from build123d import *

# Parameters (mm, degrees)
SKETCH1_R                = 50
BOSS_EXTRUDE1_DEPTH      = 70
BOSS_EXTRUDE2_REACH      = 223.642
BOSS_EXTRUDE2_END_RADIUS = 65
SKETCH2_R                = 42
SKETCH3_R                = 39.5
BOSS_EXTRUDE3_DEPTH      = 1
SKETCH6_R                = 41.25
BOSS_EXTRUDE4_DEPTH      = 1
BOSS_EXTRUDE5_START      = 7
SKETCH7_R                = 42
BOSS_EXTRUDE5_DEPTH      = 7
SKETCH8_R                = 35
BOSS_EXTRUDE6_DEPTH      = 3
SKETCH9_R                = 2.25
SKETCH9_R_2              = 1.5
BOSS_EXTRUDE8_DEPTH      = 1
CIRPATTERN1_COUNT        = 16
SKETCH10_R               = 10
BOSS_EXTRUDE9_DEPTH      = 10


with BuildPart() as part:
    # Sketch1 → Boss-Extrude1 (new, symmetric)
    with BuildSketch(Plane.XY):
        with BuildLine():
            Line((-80, -40), (-80, 40))
            Line((-80, 40), (-22.281665693, 61.061668614))
            ThreePointArc((-22.281665693, 61.061668614), (65, 0), (-22.281665693, -61.061668614))
            Line((-22.281665693, -61.061668614), (-80, -40))
        make_face()
        Circle(SKETCH1_R, mode=Mode.SUBTRACT)
    extrude(amount=BOSS_EXTRUDE1_DEPTH, both=True)

    # Boss-Extrude2: up to this cylinder (the profile starts outside it)
    boss_extrude2_end = Plane(origin=(0, 0, 0), z_dir=(0, 0, -1)) * Cylinder(BOSS_EXTRUDE2_END_RADIUS, 578.284, mode=Mode.PRIVATE)
    # Sketch2 → Boss-Extrude2 (add, up to the surface)
    with BuildSketch(Plane(origin=(120, 0, 0), x_dir=(0, 0, -1), z_dir=(1, 0, 0)), mode=Mode.PRIVATE) as boss_extrude2_sk1:
        Circle(SKETCH2_R)
    boss_extrude2_tool1 = extrude(boss_extrude2_sk1.sketch, amount=-BOSS_EXTRUDE2_REACH, mode=Mode.PRIVATE) - boss_extrude2_end
    add(boss_extrude2_tool1.solids().sort_by_distance((120, 0, 0))[0])

    # Sketch3 → Boss-Extrude3 (add)
    with BuildSketch(Plane(origin=(120, 0, 0), x_dir=(0, 0, -1), z_dir=(1, 0, 0))):
        Circle(SKETCH3_R)
    extrude(amount=BOSS_EXTRUDE3_DEPTH)

    # Sketch5 → Revolve1 (revolve)
    with BuildSketch(Plane.XY, mode=Mode.PRIVATE) as revolve1_sk:
        with BuildLine():
            Line((121, 0), (121, 40))
            ThreePointArc((121, 40), (131, 41.376973739), (141, 40))
            Line((141, 40), (141, 0))
            Line((141, 0), (121, 0))
        make_face()
    revolve(revolve1_sk.sketch.rotate(Axis((121, 0, 0), (1, 0, 0)), 90), axis=Axis((121, 0, 0), (1, 0, 0)))

    # Sketch6 → Boss-Extrude4 (add)
    with BuildSketch(Plane(origin=(141, 0, 0), x_dir=(0, 0, -1), z_dir=(1, 0, 0))):
        Circle(SKETCH6_R)
    extrude(amount=BOSS_EXTRUDE4_DEPTH)

    # Sketch7 → Boss-Extrude5 (add)
    with BuildSketch(Plane(origin=(142, 0, 0), x_dir=(0, 0, -1), z_dir=(1, 0, 0)).offset(BOSS_EXTRUDE5_START)):
        Circle(SKETCH7_R)
    boss_extrude5 = extrude(amount=-BOSS_EXTRUDE5_DEPTH)

    # Sketch8 → Boss-Extrude6 (add)
    with BuildSketch(Plane(origin=(149, 0, 0), x_dir=(0, 0, -1), z_dir=(1, 0, 0))):
        Circle(SKETCH8_R)
    extrude(amount=BOSS_EXTRUDE6_DEPTH)

    # Sketch9 → Boss-Extrude8 (add)
    with BuildSketch(Plane(origin=(149, 0, 0), x_dir=(0, 0, -1), z_dir=(1, 0, 0))):
        with Locations((38.5, 0)):
            Circle(SKETCH9_R)
        with Locations((38.5, 0)):
            Circle(SKETCH9_R_2, mode=Mode.SUBTRACT)
    boss_extrude8 = extrude(amount=BOSS_EXTRUDE8_DEPTH)

    # CirPattern1: Boss-Extrude5, Boss-Extrude8 ×16 about axis
    cirpattern1_axis = Axis((0, 0, 0), (1, 0, 0))
    add([boss_extrude5.rotate(cirpattern1_axis, i * 360 / CIRPATTERN1_COUNT) for i in range(1, CIRPATTERN1_COUNT)])
    add([boss_extrude8.rotate(cirpattern1_axis, i * 360 / CIRPATTERN1_COUNT) for i in range(1, CIRPATTERN1_COUNT)])

    # Sketch10 → Boss-Extrude9 (add)
    with BuildSketch(Plane(origin=(152, 0, 0), x_dir=(0, 0, -1), z_dir=(1, 0, 0))):
        Circle(SKETCH10_R)
    extrude(amount=BOSS_EXTRUDE9_DEPTH)


solid = part.part
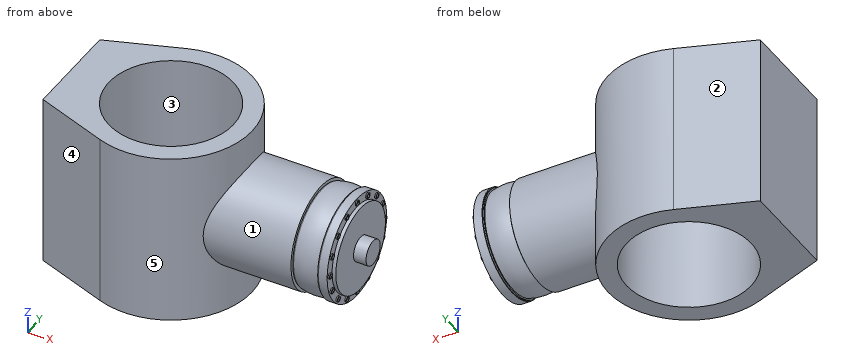
Part model, mm, in its own coordinate system. Face numbers are marked on the shaded views. A direction names the side the tool comes from. Coordinates: 2 decimals unless noted, no trailing zeros. Order: outer loops, then holes, each group sorted by start corner. A loop starts at its lowest first (then second) coordinate and runs counter-clockwise, first axis right, second up. Notation, with made-up numbers: M 52.5,47.25 L 66.5,47.25 A33 ccw 66.5,82.25 Z; hole C -11,-8 d9. An arc over 180 degrees is marked long. Use a Markdown table: item, result.
(1) Probe L1, parallel to Y at x = -39.5, z = -11; L2, parallel to Y at x = 14.5, z = 39.5; L3, parallel to X at y = -8, z = -53.5. List the from-to ranges inside material, lowest first.
A:
| item | result |
|---|---|
| L1 | y = -54.78 to -30.66, 30.66 to 54.78 |
| L2 | y = -63.36 to -47.85, 47.85 to 63.36 |
| L3 | x = -80 to -49.36, 49.36 to 64.51 |
(2) Cut at C-C on x = 98. Write the cut outline in (y, z).
A:
| item | result |
|---|---|
| outline | C 0,0 d84 |
(3) Pull direction X, two halves, no side cores. Call the marked faces 3, 4 and 5: released by +X, released by -X, zero draft, split by the parting line, or undercut.
A:
| item | result |
|---|---|
| face 3 | undercut |
| face 4 | released by -X |
| face 5 | split by the parting line |
(4) Tool access for the marked faces 1 and 2: list every direction of +Z, -Z, +X, -X, +Y, -Y with a clear straight run to the whole face (end or side of a thin tool).
A:
| item | result |
|---|---|
| face 1 | +X |
| face 2 | +Z, -Z, -X, +Y |
(5) Cut at B-B on x = 30. Write the cut outline in (y, z), then the cut area to 3 significant figures.
A:
| item | result |
|---|---|
| outline | M -57.66,-70 L -40,-70 L -40,70 L -57.66,70 Z; M 40,-70 L 57.66,-70 L 57.66,70 L 40,70 Z |
| area | 4,950 mm^2 |
(6) Cut at A-A on x = 0. Write the cut outline in (y, z).
A:
| item | result |
|---|---|
| outline | M -65,-70 L -50,-70 L -50,70 L -65,70 Z; M 50,-70 L 65,-70 L 65,70 L 50,70 Z |
(7) Flat gauge pins, fed straight in: pin 1 (3.5 mm diameter, centred on y = -35.5, z = 14.5, fed in from +X); pin 2 (4 mm diameter, centred on x = 102, y = -35.5, fed in from +Z); pin 3 (6 mm diameter, centred on y = -15.5, z = 46, fed in from +X). Where does each tip first touch, or does it go through?
A:
| item | result |
|---|---|
| pin 1 | stops at x = 150 |
| pin 2 | stops at z = 25.33 |
| pin 3 | stops at x = 63.79 |
